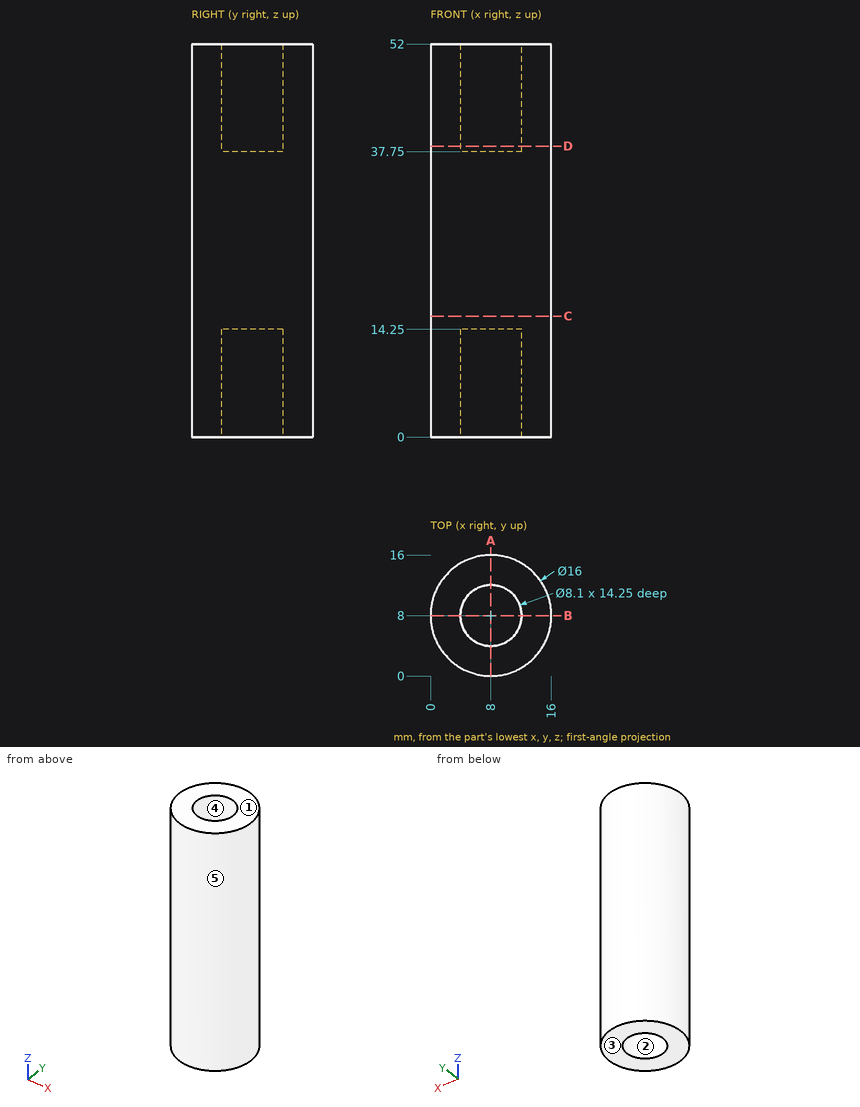
Print and shaded views of the part. All mm, measured from the part's lowest x, y and z. A direction names the side the tool comes from. Coordinates: 2 decimals unless noted, no trailing zeros. Loops run counter-clockwise (first coordinate to the right, second up) from the corner with the lowest first, then second, coordinate; pieces in that order, holes last. Notation, with made-up numbers: (34.5, 7.25) - (64.5, 7.25) arc R10 ccw to (64.5, 17.25) - close; hole circle Ø3 at (84, 16.25). An arc over 180 degrees is marked (long way). Write item = value, one per line. Start each with the question number.
Item 1: Cut at C-C, the plane z = 16. Give the cut face in (x, y), and give its area (3 significant figures).
Item 2: 3-axis set-ups, long thin cutter, end or side, ignore diameter. For the marked faces 1 and 2: which of +Z, -Z, +X, -X, +Y, -Y reach the whole face in a straight line?
Item 3: Cut at D-D, the plane z = 38.5. Give the cut face in (x, y), and give its area (3 significant figures).
Item 4: Mould opens along X. For the marked faces 3, 4 and 5 say: released by +X, released by -X, zero draft, split by the parting line, or undercut.
Item 5: Flat gauge pins, fed straight in: pin 1 Ø2 at (x, z) = (9.5, 41.5) entering from -Y; pin 2 Ø5 at (x, y) = (8, 8) entering from +Z. Where does each tip first touch, or does it go through?
Item 6: Cut at A-A, the plane x = 8. Give the cut face in (y, z).
Item 7: Wall check: L1, parallel to Y at x = 8, z = 43.75; L2, parallel to Y at x = 7.75, z = 37; L3, parallel to Z at x = 4.5, y = 6.75. Give the ranges that are in metal, low to high. Write a range as from..to.
The answers:
q1.outline = circle Ø16 at (8, 8)
q1.area = 201 mm2
q2.face_1 = +Z, +X, -X, +Y, -Y
q2.face_2 = -Z
q3.outline = circle Ø16 at (8, 8); hole circle Ø8.1 at (8, 8)
q3.area = 150 mm2
q4.face_3 = zero draft
q4.face_4 = undercut
q4.face_5 = split by the parting line
q5.pin_1 = 0.02
q5.pin_2 = 37.75
q6.outline = (0, 0) - (3.95, 0) - (3.95, 14.25) - (12.05, 14.25) - (12.05, 0) - (16, 0) - (16, 52) - (12.05, 52) - (12.05, 37.75) - (3.95, 37.75) - (3.95, 52) - (0, 52) - close
q7.L1 = 0..3.95, 12.05..16
q7.L2 = 0..16
q7.L3 = 14.25..37.75
